```python
from build123d import *

# Parameters (mm, degrees)
BOSS_EXTRUDE1_DEPTH = 10.7188
SKETCH2_OUTSIDE_W   = 36.066
SKETCH2_OUTSIDE_H   = 73.696
CUT_EXTRUDE1_DEPTH  = 60.909415415
FILLET1_R           = 2.54
SKETCH6_R           = 1.27
CUT_EXTRUDE3_DEPTH  = 60.576572944
FILLET2_R           = 2.54


with BuildPart() as part:
    # Sketch1 → Boss-Extrude1 (new, symmetric)
    with BuildSketch(Plane(origin=(0, 0, 0), x_dir=(0, 0, -1), z_dir=(1, 0, 0))):
        Polygon((-4.567857039, -57.925462145), (-0.745157039, -57.925462145), (-0.745157039, -30.364014398), (1.670365013, -30.742566651), (4.326872052, -0.378552253), (-4.326872052, 0.378552253), (-6.983379091, -29.985462145), (-4.567857039, -30.364014398), align=None)
    extrude(amount=BOSS_EXTRUDE1_DEPTH, both=True)

    # Sketch2 outside → Cut-Extrude1 (cut, through all)
    # profile 1 of 2: a face of its own
    with BuildSketch(Plane(origin=(0, 0.378552253, 4.326872052), x_dir=(1, 0, 0), z_dir=(0, 0.08715574274765905, 0.9961946980917455))):
        with Locations((0, -28.78)):
            Rectangle(SKETCH2_OUTSIDE_W, SKETCH2_OUTSIDE_H)
        with BuildLine():
            Line((5.94995, -30.48), (10.375772253, -13.408785796))
            ThreePointArc((10.375772253, -13.408785796), (0, 0), (-10.375772253, -13.408785796))
            Line((-10.375772253, -13.408785796), (-5.94995, -30.48))
            Line((-5.94995, -30.48), (-5.94995, -58.103153246))
            Line((-5.94995, -58.103153246), (5.94995, -58.103153246))
            Line((5.94995, -58.103153246), (5.94995, -30.48))
        make_face(mode=Mode.SUBTRACT)
    # profile 2 of 2: a face of its own
    with BuildSketch(Plane(origin=(0, 0.378552253, 4.326872052), x_dir=(1, 0, 0), z_dir=(0, 0.08715574274765905, 0.9961946980917455))):
        Polygon((4.648522628, -6.070277372), (1.701477372, -4.3688), (-1.701477372, -4.3688), (-4.648522628, -6.070277372), (-6.35, -9.017322628), (-6.35, -12.420277372), (-4.648522628, -15.367322628), (-1.701477372, -17.0688), (1.701477372, -17.0688), (4.648522628, -15.367322628), (6.35, -12.420277372), (6.35, -9.017322628), align=None)
    extrude(amount=-CUT_EXTRUDE1_DEPTH, mode=Mode.SUBTRACT)

    # Fillet1
    # the kernel refuses this fillet: 2.54 mm, written as the material it adds along each edge
    with BuildSketch(Plane(origin=(-13.281888943, -30.364014398, 0.745157039), x_dir=(0, -0.15482679187338919, -0.9879416301169793), z_dir=(1, 0, 0))) as fillet1_piece_1_section:
        with BuildLine():
            CenterArc((2.960769294, -2.487084038), FILLET1_R, 101.715774122, 87.190976769)
            Line((0.451397554, -2.880344089), (0.401210119, -2.88820929))
            Line((0.401210119, -2.88820929), (-0.050187435, -0.007865201))
            Line((-0.050187435, -0.007865201), (0, 0.0508))
            ThreePointArc((0, 0.0508), (1.222502412, 0.0508), (2.434689535, 0.049741681))
            Line((2.434689535, 0.049741681), (2.445004824, 0))
        make_face()
    fillet1_piece_1 = extrude(amount=26.563777885, mode=Mode.PRIVATE)
    fillet1_piece_1 = split(fillet1_piece_1, bisect_by=Plane(origin=(-5.94995, -31.737023375, 0.445932994), z_dir=(1, 0, 0)), keep=Keep.TOP, mode=Mode.PRIVATE)
    fillet1_piece_1 = split(fillet1_piece_1, bisect_by=Plane(origin=(-5.654886332, -31.700159235, 0.4427078), z_dir=(-0.9679975606806361, -0.2500046262979335, 0.021872570630104494)), keep=Keep.TOP, mode=Mode.PRIVATE)
    add(fillet1_piece_1)
    with BuildSketch(Plane(origin=(-13.281888943, -30.364014398, 0.745157039), x_dir=(0, -0.15482679187338919, -0.9879416301169793), z_dir=(1, 0, 0))) as fillet1_piece_2_section:
        with BuildLine():
            CenterArc((2.960769294, -2.487084038), FILLET1_R, 101.715774122, 87.190976769)
            Line((0.451397554, -2.880344089), (0.401210119, -2.88820929))
            Line((0.401210119, -2.88820929), (-0.050187435, -0.007865201))
            Line((-0.050187435, -0.007865201), (0, 0.0508))
            ThreePointArc((0, 0.0508), (1.222502412, 0.0508), (2.434689535, 0.049741681))
            Line((2.434689535, 0.049741681), (2.445004824, 0))
        make_face()
    fillet1_piece_2 = extrude(amount=26.563777885, mode=Mode.PRIVATE)
    fillet1_piece_2 = split(fillet1_piece_2, bisect_by=Plane(origin=(-5.94995, -31.133883126, 0.125173685), z_dir=(1, 0, 0)), keep=Keep.TOP, mode=Mode.PRIVATE)
    fillet1_piece_2 = split(fillet1_piece_2, bisect_by=Plane(origin=(5.442501536, -32.539517415, 0.248150751), z_dir=(-0.967997560680636, 0.2500046262979333, -0.021872570630104476)), keep=Keep.TOP, mode=Mode.PRIVATE)
    fillet1_piece_2 = split(fillet1_piece_2, bisect_by=Plane(origin=(-5.442501536, -32.539517415, 0.248150751), z_dir=(0.9679975606806361, 0.2500046262979335, -0.021872570630104494)), keep=Keep.TOP, mode=Mode.PRIVATE)
    fillet1_piece_2 = split(fillet1_piece_2, bisect_by=Plane(origin=(5.94995, -31.133883126, 0.125173685), z_dir=(-1, 0, 0)), keep=Keep.TOP, mode=Mode.PRIVATE)
    add(fillet1_piece_2)
    with BuildSketch(Plane(origin=(-13.281888943, -30.364014398, 0.745157039), x_dir=(0, -0.15482679187338919, -0.9879416301169793), z_dir=(1, 0, 0))) as fillet1_piece_3_section:
        with BuildLine():
            CenterArc((2.960769294, -2.487084038), FILLET1_R, 101.715774122, 87.190976769)
            Line((0.451397554, -2.880344089), (0.401210119, -2.88820929))
            Line((0.401210119, -2.88820929), (-0.050187435, -0.007865201))
            Line((-0.050187435, -0.007865201), (0, 0.0508))
            ThreePointArc((0, 0.0508), (1.222502412, 0.0508), (2.434689535, 0.049741681))
            Line((2.434689535, 0.049741681), (2.445004824, 0))
        make_face()
    fillet1_piece_3 = extrude(amount=26.563777885, mode=Mode.PRIVATE)
    fillet1_piece_3 = split(fillet1_piece_3, bisect_by=Plane(origin=(-5.94995, -30.484623478, 0.0088191), z_dir=(-1, 0, 0)), keep=Keep.TOP, mode=Mode.PRIVATE)
    fillet1_piece_3 = split(fillet1_piece_3, bisect_by=Plane(origin=(-5.977723598, -30.488093407, 0.009122679), z_dir=(0.9679975606806361, 0.2500046262979335, -0.021872570630104494)), keep=Keep.TOP, mode=Mode.PRIVATE)
    add(fillet1_piece_3)
    with BuildSketch(Plane(origin=(-13.281888943, -30.364014398, 0.745157039), x_dir=(0, -0.15482679187338919, -0.9879416301169793), z_dir=(1, 0, 0))) as fillet1_piece_4_section:
        with BuildLine():
            CenterArc((2.960769294, -2.487084038), FILLET1_R, 101.715774122, 87.190976769)
            Line((0.451397554, -2.880344089), (0.401210119, -2.88820929))
            Line((0.401210119, -2.88820929), (-0.050187435, -0.007865201))
            Line((-0.050187435, -0.007865201), (0, 0.0508))
            ThreePointArc((0, 0.0508), (1.222502412, 0.0508), (2.434689535, 0.049741681))
            Line((2.434689535, 0.049741681), (2.445004824, 0))
        make_face()
    fillet1_piece_4 = extrude(amount=26.563777885, mode=Mode.PRIVATE)
    fillet1_piece_4 = split(fillet1_piece_4, bisect_by=Plane(origin=(5.654886332, -31.700159235, 0.4427078), z_dir=(0.967997560680636, -0.2500046262979333, 0.021872570630104476)), keep=Keep.TOP, mode=Mode.PRIVATE)
    fillet1_piece_4 = split(fillet1_piece_4, bisect_by=Plane(origin=(5.94995, -31.737023375, 0.445932994), z_dir=(-1, 0, 0)), keep=Keep.TOP, mode=Mode.PRIVATE)
    add(fillet1_piece_4)
    with BuildSketch(Plane(origin=(-13.281888943, -30.364014398, 0.745157039), x_dir=(0, -0.15482679187338919, -0.9879416301169793), z_dir=(1, 0, 0))) as fillet1_piece_5_section:
        with BuildLine():
            CenterArc((2.960769294, -2.487084038), FILLET1_R, 101.715774122, 87.190976769)
            Line((0.451397554, -2.880344089), (0.401210119, -2.88820929))
            Line((0.401210119, -2.88820929), (-0.050187435, -0.007865201))
            Line((-0.050187435, -0.007865201), (0, 0.0508))
            ThreePointArc((0, 0.0508), (1.222502412, 0.0508), (2.434689535, 0.049741681))
            Line((2.434689535, 0.049741681), (2.445004824, 0))
        make_face()
    fillet1_piece_5 = extrude(amount=26.563777885, mode=Mode.PRIVATE)
    fillet1_piece_5 = split(fillet1_piece_5, bisect_by=Plane(origin=(5.977723598, -30.488093407, 0.009122679), z_dir=(-0.967997560680636, 0.2500046262979333, -0.021872570630104476)), keep=Keep.TOP, mode=Mode.PRIVATE)
    fillet1_piece_5 = split(fillet1_piece_5, bisect_by=Plane(origin=(5.94995, -30.484623478, 0.0088191), z_dir=(1, 0, 0)), keep=Keep.TOP, mode=Mode.PRIVATE)
    add(fillet1_piece_5)
    with BuildSketch(Plane(origin=(5.94995, -30.364014398, 4.567857039), x_dir=(0, 0.15482679187338733, 0.9879416301169794), z_dir=(-1, 0, 0))) as fillet1_piece_6:
        with BuildLine():
            CenterArc((FILLET1_R * 0.855489011053, -FILLET1_R), FILLET1_R, 90, 81.093249109)
            Line((-FILLET1_R * 0.132452619064, -FILLET1_R * 0.845173208127), (-FILLET1_R * 0.152211451667, -FILLET1_R * 0.842076672289))
            Line((-FILLET1_R * 0.152211451667, -FILLET1_R * 0.842076672289), (-FILLET1_R * 0.0171097802211, FILLET1_R * 0.02))
            Line((-FILLET1_R * 0.0171097802211, FILLET1_R * 0.02), (FILLET1_R * 0.855489011053, FILLET1_R * 0.02))
            Line((FILLET1_R * 0.855489011053, FILLET1_R * 0.02), (FILLET1_R * 0.855489011053, 0))
        make_face()
    extrude(amount=11.8999)

    # Sketch6 → Cut-Extrude3 (cut, through all)
    with BuildSketch(Plane.XY.offset(4.567857039)):
        with Locations((0, -49.046956486)):
            Circle(SKETCH6_R)
    extrude(amount=-CUT_EXTRUDE3_DEPTH, mode=Mode.SUBTRACT)

    # Fillet2
    fillet2_edges = [part.edges().sort_by_distance(p)[0] for p in [
        (5.94995, -57.925462145, 2.656507039),
        (-5.94995, -57.925462145, 2.656507039),
    ]]
    fillet(fillet2_edges, radius=FILLET2_R)


solid = part.part
```
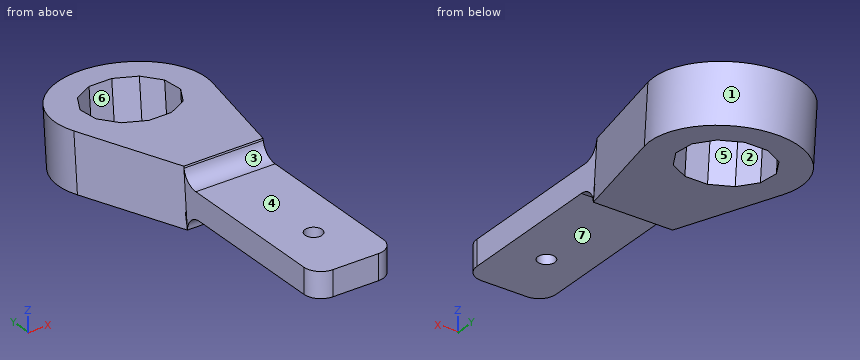
Verification items for the finished model (mm, model axes). Face numbers are marked on the shaded views. A direction names the side the tool comes from. Give positions to 0.01 mm unless a question says otherwise; leave off trailing zeros. Loops run counter-clockwise (first coordinate to the right, second up) from the corner with the lowest first, then second, coordinate; pieces in that order, holes last.
1. Section check D-D, the plane z = 2. Count the separate pieces of the cut face and the enclosed holes in it, then the cut area to 3 significant figures.
2. Section check C-C, the plane y = -40. Enter the section's corners in (x, z).
3. Mould release check, pull along X, two halves, no side actions. Record for the marked faces 1, 2 and 3: released by +X, released by -X, zero draft, split by the parting line, or undercut.
4. Go/stop test with flat-tipped pins: pin 1 Ø9.5 at (x, y) = (-0.5, -43) entering from +Z; pin 2 Ø1 at (y, z) = (-50.5, 2.5) entering from +X; pin 3 Ø5 at (y, z) = (-30, 5) entering from +X; pin 4 Ø3.5 at (y, z) = (-11.5, 1.5) entering from -X. Record where each tip stops, or that it passes through.
5. Section check B-B, the plane x = 2.75. Enter the section's corners in (y, z), then the cut area to 3 significant figures.
6. Set-up check for the marked faces 4, 5, 6 and 7: record each of +Z, -Z, +X, -X, +Y, -Y from which the full face is reachable in a straight line by a thin tool's end or side.
7. Thickness scan on line 1 (Z direction, x = -5.25, y = -38); line 2 (X direction, y = -52, z = 4.25); line 3 (Y direction, x = 4, z = 4.25). Record the ranges inside material, lowest first.
8. Section check A-A, the plane x = 0. Enter the section's corners in (y, z), then the cut area to 3 significant figures.
Geometry says:
1. separate pieces: 1
1. enclosed holes: 2
1. area: 708 mm2
2. outline: (-5.95, 0.75) - (5.95, 0.75) - (5.95, 4.57) - (-5.95, 4.57) - close
3. face 1: split by the parting line
3. face 2: undercut
3. face 3: zero draft
4. pin 1: stops at z = 4.57
4. pin 2: stops at x = 5.95
4. pin 3: stops at x = 6.64
4. pin 4: stops at x = -10.72
5. outline: (-57.93, 0.75) - (-33.28, 0.75) arc R2.54 cw to (-30.74, -1.67) - (-16.78, -2.89) - (-16.02, 5.76) - (-29.99, 6.98) - (-30.03, 6.71) arc R2.54 cw to (-32.54, 4.57) - (-57.93, 4.57) - close; (-5.33, -3.89) - (-0.74, -4.3) - (0.02, 4.36) - (-4.58, 4.76) - close
5. area: 270 mm2
6. face 4: +Z, +X, -X, -Y
6. face 5: -Z
6. face 6: +Z
6. face 7: -Z, +X, -X, -Y
7. line 1: z = 0.75 to 4.57
7. line 2: x = -5.95 to 5.95
7. line 3: y = -57.86 to -15.43, -5.35 to -0.41
8. outline: (-57.93, 0.75) - (-50.32, 0.75) - (-50.32, 4.57) - (-57.93, 4.57) - close; (-47.78, 0.75) - (-33.28, 0.75) arc R2.54 cw to (-30.74, -1.67) - (-17.38, -2.84) - (-16.63, 5.81) - (-29.99, 6.98) - (-30.03, 6.71) arc R2.54 cw to (-32.54, 4.57) - (-47.78, 4.57) - close; (-4.73, -3.95) - (-0.38, -4.33) - (0.38, 4.33) - (-3.97, 4.71) - close
8. area: 253 mm2
